from build123d import *

# Parameters (mm, degrees)
PAD001_DEPTH = 10
FILLET001_R  = 6
FILLET002_R  = 1


with BuildPart() as part:
    # Sketch002 → Pad001 (new body)
    with BuildSketch(Plane.XY):
        with BuildLine():
            Line((60, 64), (0, 64))
            ThreePointArc((0, 64), (-63.999936, 0), (0, -64))
            Line((60, -64), (0, -64))
            Line((60, -62), (60, -64))
            Line((0, -62), (60, -62))
            ThreePointArc((0, 62), (-61.999985, 0), (0, -62))
            Line((0, 62), (60, 62))
            Line((60, 64), (60, 62))
        make_face()
    extrude(amount=PAD001_DEPTH)

    # Fillet001
    fillet001_edges = [part.edges().sort_by_distance(p)[0] for p in [
        (60, -63, 10),
        (60, 63, 10),
    ]]
    fillet(fillet001_edges, radius=FILLET001_R)

    # Fillet002
    fillet002_edges = [part.edges().sort_by_distance(p)[0] for p in [
        (27, 64, 10),
    ]]
    fillet(fillet002_edges, radius=FILLET002_R)


solid = part.part
Model file for the job. Use its own axes, mm. A direction names the side the tool comes from. Give positions to 0.01 mm unless a question says otherwise; leave off trailing zeros. Loops run counter-clockwise (first coordinate to the right, second up) from the corner with the lowest first, then second, coordinate; pieces in that order, holes last. Notation, with made-up numbers: (16, 67.5) - (71, 67.5) arc R16 ccw to (71, 95.5) - close; hole circle Ø9 at (67.5, 39.25). An arc over 180 degrees is marked (long way). Use one line per item in the form item = value.
(1) Drop flat-ended pins along their axis: P1, Ø4, axis at y = -13.5, z = 4, coming from the -X side; P2, Ø6, axis at y = -6.5, z = 9, coming from the +X side. Give the stop position or say it passes through.
Determined:
P1 = -62.96
P2 = -61.27
(2) Cut at B-B (z = 2). Give the cut face in (x, y), then the cut area to 3 significant figures.
Determined:
outline = (0, -64) - (59, -64) arc R1 ccw to (60, -63) - (60, -62) - (0, -62) arc R62 cw to (0, 62) - (60, 62) - (60, 63) arc R1 ccw to (59, 64) - (0, 64) arc R64 ccw to start
area = 635 mm^2
(3) Cut at A-A (x = 35). Give the cut face in (y, z).
Determined:
outline = (-64, 0) - (-62, 0) - (-62, 10) - (-63, 10) arc R1 ccw to (-64, 9) - close; (62, 0) - (64, 0) - (64, 9) arc R1 ccw to (63, 10) - (62, 10) - close
(4) 3-axis set-ups, long thin cutter, end or side, ignore diameter. For faces 5 (the face through (30, -62, 5)), 6 (the face through (-63.984, 1.407, 4.437)): which of +Z, -Z, +X, -X, +Y, -Y reach the whole face in a straight line?
Determined:
face_5 = +Z, -Z, +X
face_6 = +Z, -Z, -X
(5) Drill centre lines: L1, parallel to Y at x = 20, z = 2.5; L2, parallel to Y at x = -57, z = 7; L3, parallel to X at y = 15, z = 8. Where is each one in solid material? Low to high.
Determined:
L1 = -64 to -62, 62 to 64
L2 = -29.1 to -24.39, 24.39 to 29.1
L3 = -62.22 to -60.16
(6) Cut at C-C (y = 0). Give the cut face in (x, z), then the cut area to 3 significant figures.
Determined:
outline = (-64, 0) - (-62, 0) - (-62, 10) - (-63, 10) arc R1 ccw to (-64, 9) - close
area = 19.8 mm^2
(7) Pull direction Y, two halves, no side cores. Call faces 1 (the face through (-61.985, 1.363, 4.93)), 2 (the face through (-62, 5, 0)), 3 (the face through (30, 62, 5)), 4 (the face through (30, 64, 4)): pulls with the +Y half, pulls with the -Y half, needs draft (parallel to the pull), parting line crosses it, or undercut.
Determined:
face_1 = undercut
face_2 = needs draft
face_3 = undercut
face_4 = pulls with the +Y half
